Build history of the part. All positions in model axes, mm. A direction names the side the tool comes from. Give positions to 0.01 mm unless a question says otherwise; leave off trailing zeros. Loops run counter-clockwise (first coordinate to the right, second up) from the corner with the lowest first, then second, coordinate; pieces in that order, holes last.
1) Two-plate mould, pull along Z, no slides. Class faces 3 (the cylindrical face through (0, 3, 15)), 4 (the flat face through (-3, 26.4, 3)), 5 (the cylindrical face through (0.33, 16.057, -7.493)): +Z half, -Z half, draft (parallel to the pull), parting line (faces both ways), or undercut.
2) Wall check: line 1 (Y direction, x = -10.5, z = 7.5); line 2 (Z direction, x = 2, y = 2.25); line 3 (X direction, y = 9.5, z = 0). Give the ranges that are in metal, low to high.
3) Band-saw the part on A-A on x = -14. List the corners of the cut face in (y, z).
4) Flat gauge pins, fed straight in: P1, Ø12, axis at x = -6.5, z = -12, coming from the +Y side; P2, Ø10, axis at x = -7.5, y = 9.5, coming from the -Z side; P3, Ø3, axis at y = 17.5, z = -4.5, coming from the -X side. Where does each tip first touch, or does it go through?
5) Band-saw the part on D-D on y = 10. List the corners of the cut face in (x, z).
6) Band-saw the part on B-B on x = 0. List the corners of the cut face in (y, z).
7) 3-axis set-ups, long thin cutter, end or side, ignore diameter. For faces 1 (the cylindrical face through (15, 3, 0)), 2 (the flat face through (-8, 6, 0)): which of +Z, -Z, +X, -X, +Y, -Y reach the whole face in a straight line?
8) Band-saw the part on C-C on z = -3. List the corners of the cut face in (x, y), then the cut area to 3 significant figures.
```python
from build123d import *

# Parameters (mm, degrees)
SKETCH_1_R               = 17.5
EXTRUDE_1_DEPTH          = 6
SKETCH_3_R               = 7.5
EXTRUDE_2_DEPTH          = 20.4
SKETCH_4_R               = 4
CUT_EXTRUDE_1_DEPTH      = 37.186461557
SKETCH_5_R               = 2.5
CUT_EXTRUDE_2_DEPTH      = 10
PATTERN_CIRCULAR_1_COUNT = 4


with BuildPart() as part:
    # 草图1 → 凸台-拉伸1 (new body)
    with BuildSketch(Plane(origin=(0, 0, 0), x_dir=(1, 0, 0), z_dir=(0, 1, 0))):
        with Locations(Location((0, 0, 0), (0, 0, 270))):
            Circle(SKETCH_1_R)
    extrude(amount=EXTRUDE_1_DEPTH)

    # 草图3 → 凸台-拉伸2 (add)
    with BuildSketch(Plane(origin=(0, 6, 0), x_dir=(1, 0, 0), z_dir=(0, 1, 0))):
        with Locations(Location((0, 0, 0), (0, 0, 270))):
            Circle(SKETCH_3_R)
    extrude(amount=EXTRUDE_2_DEPTH)

    # 草图4 → 切除-拉伸1 (cut, through all)
    with BuildSketch(Plane(origin=(0, 26.4, 0), x_dir=(1, 0, 0), z_dir=(0, 1, 0))):
        with Locations(Location((0, 0, 0), (0, 0, 270))):
            Circle(SKETCH_4_R)
    extrude(amount=-CUT_EXTRUDE_1_DEPTH, mode=Mode.SUBTRACT)

    # 草图5 → 切除-拉伸2 (cut)
    with BuildSketch(Plane(origin=(0, 6, 0), x_dir=(1, 0, 0), z_dir=(0, 1, 0))):
        with Locations(Location((0, 12.5, 0), (0, 0, 270))):
            Circle(SKETCH_5_R)
    cut_extrude_2 = extrude(amount=-CUT_EXTRUDE_2_DEPTH, mode=Mode.SUBTRACT)

    # 阵列(圆周)1: 切除-拉伸2 ×4 about axis
    pattern_circular_1_axis = Axis((0, 0, 0), (0, 1, 0))
    for i in range(1, PATTERN_CIRCULAR_1_COUNT):
        add(cut_extrude_2.rotate(pattern_circular_1_axis, i * 360 / PATTERN_CIRCULAR_1_COUNT), mode=Mode.SUBTRACT)


solid = part.part
```
Findings below:
1. face 3: undercut
1. face 4: draft
1. face 5: parting line
2. line 1: y = 0 to 6
2. line 2: z = -17.39 to -14, -11 to -3.46, 3.46 to 11, 14 to 17.39
2. line 3: x = -7.5 to -4, 4 to 7.5
3. outline: (0, -10.5) - (6, -10.5) - (6, -2) - (0, -2) - close; (0, 2) - (6, 2) - (6, 10.5) - (0, 10.5) - close
4. P1: stops at y = 6
4. P2: stops at z = -17.05
4. P3: stops at x = -6.87
5. outline: circle Ø15 at (0, 0); hole circle Ø8 at (0, 0)
6. outline: (0, -17.5) - (6, -17.5) - (6, -15) - (0, -15) - close; (0, -10) - (6, -10) - (6, -7.5) - (26.4, -7.5) - (26.4, -4) - (0, -4) - close; (0, 4) - (26.4, 4) - (26.4, 7.5) - (6, 7.5) - (6, 10) - (0, 10) - close; (0, 15) - (6, 15) - (6, 17.5) - (0, 17.5) - close
7. face 1: +Y, -Y
7. face 2: +Y
8. outline: (-17.24, 0) - (-2.65, 0) - (-2.65, 26.4) - (-6.87, 26.4) - (-6.87, 6) - (-17.24, 6) - close; (2.65, 0) - (17.24, 0) - (17.24, 6) - (6.87, 6) - (6.87, 26.4) - (2.65, 26.4) - close
8. area: 348 mm2
